The model under review builds one solid part; all positions refer to its coordinate system, in mm. A direction names the side the tool comes from. Give positions to 0.01 mm unless a question says otherwise; leave off trailing zeros. Loops run counter-clockwise (first coordinate to the right, second up) from the corner with the lowest first, then second, coordinate; pieces in that order, holes last. Notation, with made-up numbers: (-29, 58) - (26, 58) arc R23 ccw to (26, 75) - close; hole circle Ø11 at (-7.75, -23). An arc over 180 degrees is marked (long way). Return JSON: item names as keys, results as strings. Group by question number.
from build123d import *

# Parameters (mm, degrees)
Y_KSEKLIK_EKSTR_ZYON1_DEPTH = 400
Y_KSEKLIK_EKSTR_ZYON3_DEPTH = 40
Y_KSEKLIK_EKSTR_ZYON4_DEPTH = 360
IZIM16_R                    = 20
Y_KSEKLIK_EKSTR_ZYON5_DEPTH = 10
IZIM17_R                    = 8
KES_EKSTR_ZYON21_DEPTH      = 50
IZIM19_W                    = 11.493054453
IZIM19_H                    = 360
KES_EKSTR_ZYON23_DEPTH      = 170
KES_EKSTR_ZYON24_DEPTH      = 170


# Read off the part's stored shape, not the designer's step: Kubbe1
with BuildPart() as part:
    # Çizim1 → Yükseklik-Ekstrüzyon1 (new body)
    with BuildSketch(Plane(origin=(0, 0, 0), x_dir=(1, 0, 0), z_dir=(0, 1, 0))):
        with BuildLine():
            Line((0, 140), (0, 100))
            ThreePointArc((0, 100), (100, 0), (0, -100))
            Line((0, -100), (0, -140))
            ThreePointArc((0, -140), (140, 0), (0, 140))
        make_face()
    extrude(amount=-Y_KSEKLIK_EKSTR_ZYON1_DEPTH)

    # Çizim2 → Yükseklik-Ekstrüzyon3 (add)
    with BuildSketch(Plane(origin=(0, 0, 0), x_dir=(1, 0, 0), z_dir=(0, 1, 0))):
        with BuildLine():
            Line((59.548618827, 126.704230378), (290.629357971, 18.10060434))
            ThreePointArc((290.629357971, 18.10060434), (302.122412424, 0), (290.629357971, -18.10060434))
            Line((290.629357971, -18.10060434), (59.548618827, -126.704230378))
            ThreePointArc((59.548618827, -126.704230378), (30.507439642, -136.635632712), (0, -140))
            Line((0, -140), (0, -100))
            ThreePointArc((0, -100), (100, 0), (0, 100))
            Line((0, 100), (0, 140))
            ThreePointArc((0, 140), (30.507439642, 136.635632712), (59.548618827, 126.704230378))
        make_face()
    extrude(amount=-Y_KSEKLIK_EKSTR_ZYON3_DEPTH)

    # Çizim5 → Yükseklik-Ekstrüzyon4 (add)
    with BuildSketch(Plane(origin=(0, -40, 0), x_dir=(1, 0, 0), z_dir=(0, 1, 0))):
        with BuildLine():
            Line((290.629357971, 18.10060434), (98.34819837, 18.10060434))
            ThreePointArc((98.34819837, 18.10060434), (100, 0), (98.34819837, -18.10060434))
            Line((98.34819837, -18.10060434), (290.629357971, -18.10060434))
            ThreePointArc((290.629357971, -18.10060434), (302.122412424, 0), (290.629357971, 18.10060434))
        make_face()
    extrude(amount=-Y_KSEKLIK_EKSTR_ZYON4_DEPTH)

    # Çizim16 → Yükseklik-Ekstrüzyon5 (add)
    with BuildSketch(Plane(origin=(0, 0, 0), x_dir=(1, 0, 0), z_dir=(0, 1, 0))):
        with Locations(Location((270, 0, 0), (0, 0, 270))):
            Circle(IZIM16_R)
    extrude(amount=Y_KSEKLIK_EKSTR_ZYON5_DEPTH)

    # Kubbe1 outline → Kubbe1 (revolve)
    with BuildSketch(Plane(origin=(270, 0, 0), x_dir=(1, 0, 0), z_dir=(0, 0, 1))):
        with BuildLine():
            Line((0, 10), (20.000000025, 9.99999998))
            ThreePointArc((20.000000025, 9.99999998), (10.594810065, 15.199457281), (0, 17))
            Line((0, 17), (0, 10))
        make_face()
    revolve(axis=Axis((270, 0, 0), (0, 1, 0)))

    # Çizim17 → Kes-Ekstrüzyon21 (cut)
    with BuildSketch(Plane.ZY):
        with Locations((120, -50)):
            Circle(IZIM17_R)
        with Locations((120, -110)):
            Circle(IZIM17_R)
        with Locations((120, -170)):
            Circle(IZIM17_R)
        with Locations((120, -230)):
            Circle(IZIM17_R)
        with Locations((120, -290)):
            Circle(IZIM17_R)
        with Locations((120, -350)):
            Circle(IZIM17_R)
        with Locations(Location((-120, -350, 0), (0, 0, 180))):
            Circle(IZIM17_R)
        with Locations(Location((-120, -290, 0), (0, 0, 180))):
            Circle(IZIM17_R)
        with Locations(Location((-120, -230, 0), (0, 0, 180))):
            Circle(IZIM17_R)
        with Locations(Location((-120, -170, 0), (0, 0, 180))):
            Circle(IZIM17_R)
        with Locations(Location((-120, -110, 0), (0, 0, 180))):
            Circle(IZIM17_R)
        with Locations(Location((-120, -50, 0), (0, 0, 180))):
            Circle(IZIM17_R)
    extrude(amount=-KES_EKSTR_ZYON21_DEPTH, mode=Mode.SUBTRACT)

    # Çizim19 → Kes-Ekstrüzyon23 (cut)
    with BuildSketch(Plane.XY.offset(18.10060434)):
        with Locations((296.375885197, -220)):
            Rectangle(IZIM19_W, IZIM19_H)
    extrude(amount=-KES_EKSTR_ZYON23_DEPTH, mode=Mode.SUBTRACT)

    # Çizim21 → Kes-Ekstrüzyon24 (cut)
    with BuildSketch(Plane.XY.offset(18.10060434)):
        Polygon((290.629357971, -40), (176.145834142, -400), (290.629357971, -400), align=None)
    extrude(amount=-KES_EKSTR_ZYON24_DEPTH, mode=Mode.SUBTRACT)


solid = part.part
Item 1: Take a section at D-D (x = 270). State the section outline as (y, z) points, then the cut area to 3 significant figures.
Item 2: Mouldability with a two-part tool opening along Z and no side actions: class faces 4 (the face through (50, -110, 120)), 5 (the face through (0, -197, -120)), 6 (the face through (176.71, -19.72, 71.64)) as +Z half, -Z half, draft (parallel to the pull), parting line (faces both ways), or undercut.
Item 3: Tool access review of faces 1 (the face through (176, -40, 48)), 2 (the face through (50, -230, -120)), 3 (the face through (176, -40, -53)): name each direction out of +Z, -Z, +X, -X, +Y, -Y from which nothing blocks a thin tool from reaching the whole face with its end or side.
Item 4: For P1, Ø3, axis at y = -245.5, z = -15, coming from the -X side; P2, Ø9.5, axis at y = -50, z = 120, coming from the -X side; P3, Ø12, axis at x = 174, z = 37.5, coming from the -Y side, all flat-tipped, find the tip position at first contact; note any pin that passes through.
Item 5: Take a section at A-A (x = 22). State how many separate pieces and enclosed holes the cut face has, then the cut area to 3 significant figures.
Item 6: For L1, parallel to Y at x = 152, z = 61; L2, parallel to Z at x = 176.5, y = -315; L3, parallel to Z at x = 51, y = -93, list the stretches that pass through material, from the lowest coordinate up. Write a range as from..to.
Item 7: Take a section at B-B (y = -290). State the section outline as (x, z) points.
Check sheet entries:
{
 "1": {"outline": "(-104.87, -18.1) - (-40, -18.1) - (-40, -27.8) - (0, -27.8) - (0, -20) - (10, -20) arc R32.07 ccw to (10, 20) - (0, 20) - (0, 27.8) - (-40, 27.8) - (-40, 18.1) - (-104.87, 18.1) - close", "area": "5,160 mm^2"},
 "2": {"face 4": "undercut", "face 5": "draft", "face 6": "+Z half"},
 "3": {"face 1": "+Z, +X, -Y", "face 2": "-X", "face 3": "-Z, +X, -Y"},
 "4": {"P1": "stops at x = 98.63", "P2": "stops at x = 50", "P3": "stops at y = -40"},
 "5": {"separate pieces": "2", "enclosed holes": "12", "area": "30,200 mm^2"},
 "6": {"L1": "y = -40..0", "L2": "z = -18.1..18.1", "L3": "z = -130.38..-86.02, 86.02..130.38"},
 "7": {"outline": "(0, -140) arc R140 ccw to (138.82, -18.1) - (211.13, -18.1) - (211.13, 18.1) - (138.82, 18.1) arc R140 ccw to (0, 140) - (0, 128) - (50, 128) - (50, 112) - (0, 112) - (0, 100) arc R100 cw to (0, -100) - (0, -112) - (50, -112) - (50, -128) - (0, -128) - close"}
}
